Geometry check sheet. Reference: the model listing, model coordinates, mm. Coordinates: 2 decimals unless noted, no trailing zeros. Write each loop counter-clockwise with the first axis right and the second up, starting at its lowest first coordinate (ties: lowest second). Pieces come first, ordered by that corner, then holes. Notation, with made-up numbers: M 83.25,2.5 L 126.25,2.5 A23 ccw 126.25,20.5 Z; hole C 33.5,2.25 d11. An arc over 180 degrees is marked long. Put each result on its own line as item: value. Start each with the question number.
1) Cross-section at A-A on z = 0. Record the cut outline in (x, y).
2) Gauge pin test, flat ends, axial feed: pin 1 (5 mm diameter, centred on y = -5, z = -6.5, fed in from +X); pin 2 (6 mm diameter, centred on y = -4.5, z = 24.5, fed in from +X); pin 3 (5 mm diameter, centred on x = 17, y = -8, fed in from +Z); pin 4 (8 mm diameter, centred on x = 21, z = 19.5, fed in from +Y). Record the tip position at first contact, or that the pin passes through.
3) Cross-section at B-B on x = 0. Record the cut outline in (y, z), plus the area to 3 significant figures.
4) Scan lines: line 1 along Z through (x, y) = (0, -3.25); line 2 along X through (y, z) = (-9.75, 6.5); line 3 along Z through (x, y) = (18, -8). Record each from-to range of solid material in increasing order.
5) Mould release check, pull along Z, two halves, no side actions. Record for faces 1 (the cylindrical face through (-29.243, -5.643, -22.423)), 2 (the flat face through (19, 0, -30)), 3 (the cylindrical face through (15.85, -5.643, -30.474)): released by +Z, released by -Z, zero draft, split by the parting line, or undercut.
6) Cross-section at C-C on y = -2.75. Record the cut outline in (x, z), plus the area to 3 significant figures.
from build123d import *

# Parameters (mm, degrees)
F0_R     = 36.85
F0_R_2   = 34.35
F1_DEPTH = 12
F2_R     = 0.965685
F3_R     = 0.4


with BuildPart() as f1:
    # F0 (on Front) → F1 (new body)
    with BuildSketch(Plane.XZ):
        Circle(F0_R)
        Circle(F0_R_2, mode=Mode.SUBTRACT)
    extrude(amount=F1_DEPTH)

    # F2
    f2_edges = [f1.edges().sort_by_distance(p)[0] for p in [
        (-34.35, -12, 0),
        (-36.85, -12, 0),
    ]]
    fillet(f2_edges, radius=F2_R)

    # F3
    f3_edges = [f1.edges().sort_by_distance(p)[0] for p in [
        (-34.35, 0, 0),
        (-36.85, 0, 0),
    ]]
    fillet(f3_edges, radius=F3_R)


solid = f1.part
Answer key:
1. outline: M -36.85,-11.03 A0.97 ccw -35.88,-12 L -35.32,-12 A0.97 ccw -34.35,-11.03 L -34.35,-0.4 A0.4 ccw -34.75,0 L -36.45,0 A0.4 ccw -36.85,-0.4 Z; M 34.35,-11.03 A0.97 ccw 35.32,-12 L 35.88,-12 A0.97 ccw 36.85,-11.03 L 36.85,-0.4 A0.4 ccw 36.45,0 L 34.75,0 A0.4 ccw 34.35,-0.4 Z
2. pin 1: stops at x = 36.63
2. pin 2: stops at x = 29.93
2. pin 3: stops at z = 33.88
2. pin 4: passes through
3. outline: M -12,-35.88 A0.97 ccw -11.03,-36.85 L -0.4,-36.85 A0.4 ccw 0,-36.45 L 0,-34.75 A0.4 ccw -0.4,-34.35 L -11.03,-34.35 A0.97 ccw -12,-35.32 Z; M -12,35.32 A0.97 ccw -11.03,34.35 L -0.4,34.35 A0.4 ccw 0,34.75 L 0,36.45 A0.4 ccw -0.4,36.85 L -11.03,36.85 A0.97 ccw -12,35.88 Z
3. area: 59.1 mm²
4. line 1: z = -36.85 to -34.35, 34.35 to 36.85
4. line 2: x = -36.27 to -33.73, 33.73 to 36.27
4. line 3: z = -32.15 to -29.26, 29.26 to 32.15
5. face 1: split by the parting line
5. face 2: zero draft
5. face 3: undercut
6. outline: C 0,0 d73.7; hole C 0,0 d68.7
6. area: 559 mm²
